Geometry check sheet. Reference: the model listing, model coordinates, mm. Coordinates: 2 decimals unless noted, no trailing zeros. Write each loop counter-clockwise with the first axis right and the second up, starting at its lowest first coordinate (ties: lowest second). Pieces come first, ordered by that corner, then holes. Notation, with made-up numbers: (-28, -1.75) -> (7, -1.75) arc R19 cw to (7, 33.25) -> close; hole circle Ø7 at (47.25, -4). An arc over 180 degrees is marked (long way). Answer in a Markdown table with one row per item. Add a question column.
1. Scan lines: L1, parallel to X at y = -1.5, z = 1443; L2, parallel to Y at x = -8.5, z = 265.5; L3, parallel to X at y = 11.75, z = 1087. Record each from-to range of solid material in increasing order. Write a range as from..to.
2. Mould release check, pull along Y, two halves, no side actions. Record for faces 1 (the flat face through (0, 11, 900)), 2 (the flat face through (0, 12.5, 900)), 3 (the flat face through (0, -12.5, 900)): pulls with the +Y half, pulls with the -Y half, needs draft (parallel to the pull), parting line crosses it, or undercut.
3. Depth check by flat-ended pin: P1, Ø10, axis at x = 5.5, y = 2.5, coming from the -Z side. Enter the tip coordinate at first touch or a pass-through.
4. Cross-section at C-C on z = 316.5. Record the cut outline in (x, y), and give its area (3 significant figures).
5. Cross-section at B-B on y = -5. Record the cut outline in (x, z), and give its area (4 significant figures).
6. Cross-section at A-A on x = 14. Record the cut outline in (y, z), and give its area (4 significant figures).
```python
from build123d import *

# Parameters (mm, degrees)
F1_DEPTH = 1825


with BuildPart() as f1:
    # F0 (on Top) → F1 (new body)
    with BuildSketch(Plane.XY):
        with BuildLine():
            ThreePointArc((25, 10), (24.267767, 11.767767), (22.5, 12.5))
            Line((22.5, 12.5), (-22.5, 12.5))
            ThreePointArc((-22.5, 12.5), (-24.267767, 11.767767), (-25, 10))
            Line((-25, 10), (-25, -10))
            ThreePointArc((-25, -10), (-24.267767, -11.767767), (-22.5, -12.5))
            Line((-22.5, -12.5), (22.5, -12.5))
            ThreePointArc((22.5, -12.5), (24.267767, -11.767767), (25, -10))
            Line((25, -10), (25, 10))
        make_face()
        with BuildLine():
            ThreePointArc((23.5, -10), (23.207107, -10.707107), (22.5, -11))
            Line((22.5, -11), (-22.5, -11))
            ThreePointArc((-22.5, -11), (-23.207107, -10.707107), (-23.5, -10))
            Line((-23.5, -10), (-23.5, 10))
            ThreePointArc((-23.5, 10), (-23.207107, 10.707107), (-22.5, 11))
            Line((-22.5, 11), (23.5, 11))
            Line((23.5, 11), (23.5, -10))
        make_face(mode=Mode.SUBTRACT)
    extrude(amount=F1_DEPTH)


solid = f1.part
```
Results found:
| question | item | result |
|---|---|---|
| 1 | L1 | x = -25..-23.5, 23.5..25 |
| 1 | L2 | y = -12.5..-11, 11..12.5 |
| 1 | L3 | x = -24.29..24.29 |
| 2 | face 1 | undercut |
| 2 | face 2 | pulls with the +Y half |
| 2 | face 3 | pulls with the -Y half |
| 3 | P1 | passes through |
| 4 | outline | (-25, -10) arc R2.5 ccw to (-22.5, -12.5) -> (22.5, -12.5) arc R2.5 ccw to (25, -10) -> (25, 10) arc R2.5 ccw to (22.5, 12.5) -> (-22.5, 12.5) arc R2.5 ccw to (-25, 10) -> close; hole (-23.5, -10) arc R1 ccw to (-22.5, -11) -> (22.5, -11) arc R1 ccw to (23.5, -10) -> (23.5, 11) -> (-22.5, 11) arc R1 ccw to (-23.5, 10) -> close |
| 4 | area | 211 mm^2 |
| 5 | outline | (-25, 0) -> (-23.5, 0) -> (-23.5, 1825) -> (-25, 1825) -> close; (23.5, 0) -> (25, 0) -> (25, 1825) -> (23.5, 1825) -> close |
| 5 | area | 5,475 mm^2 |
| 6 | outline | (-12.5, 0) -> (-11, 0) -> (-11, 1825) -> (-12.5, 1825) -> close; (11, 0) -> (12.5, 0) -> (12.5, 1825) -> (11, 1825) -> close |
| 6 | area | 5,475 mm^2 |
